Autodesk Inventor part; units mm, degrees
ref_plane "YZ Plane" through (0, 0, 0) normal (1, 0, 0) x (0, 1, 0)
ref_plane "XZ Plane" through (0, 0, 0) normal (0, 1, 0) x (-1, 0, 0)
ref_plane "XY Plane" through (0, 0, 0) normal (0, 0, 1) x (1, 0, 0)
sketch "スケッチ1" plane through (0, 0, 0) normal (0, 0, 1) x (1, 0, 0)
  circle A0 centre (0, 0) radius 3
  circle A1 centre (0, 0) radius 1.25
  dimension "d0" = 6
  dimension "d1" = 2.5
extrude "押し出し1" add sketch "スケッチ1" along normal blind 50 contours A0 | A1
sketch "スケッチ2" plane through (0, 0, 50) normal (0, 0, 1) x (1, 0, 0)
  circle A0 centre (0, 0) radius 3
  circle A1 centre (0, 0) radius 1.25
  dimension "d4" = 2.5
extrude "押し出し2" cut sketch "スケッチ2" against normal blind 5 contours A1
extrude "押し出し3" cut sketch "スケッチ1" along normal blind 5 contours A1
properties part number "50mm" material "アルミニウム 2014-T4"
Geometry check sheet. Reference: the model listing, model coordinates, mm. A direction names the side the tool comes from. Give positions to 0.01 mm unless a question says otherwise; leave off trailing zeros. Write each loop counter-clockwise with the first axis right and the second up, starting at its lowest first coordinate (ties: lowest second). Pieces come first, ordered by that corner, then holes. Notation, with made-up numbers: M 40,-17 L 99,-17 A16 cw 99,-3 Z; hole C 67,21 d3. An arc over 180 degrees is marked long. Answer as CSV lines item,"result". Start each with the question number.
Q1. Section check C-C, the plane z = 10.5. Record the cut outline in (x, y).
Q2. Section check D-D, the plane y = 2.05. Record the cut outline in (x, z), then the cut area to 3 significant figures.
Q3. Material ranges on L1, parallel to Y at x = 0, z = 46.8; L2, parallel to Z at x = 0, y = 0.1; L3, parallel to Y at x = 0.1, z = 12, recorded low to high.
Q4. Release check for a two-part mould opening along Y. For faces 1 (the face through (-3, 0, 25)), 2 (the face through (-0.27, 1.22, 2.46)), 3 (the face through (1, -1, 0)) record: pulls with the +Y half, pulls with the -Y half, needs draft (parallel to the pull), parting line crosses it, or undercut.
Q5. Section check A-A, the plane x = 0. Record the cut outline in (y, z).
Q6. Tool access check on faces 4 (the face through (-0.27, -1.22, 47.54)), 5 (the face through (1, -1, 50)), 6 (the face through (0, 0, 5)). Record the directions out of +Z, -Z, +X, -X, +Y, -Y that give a thin tool (end or side, any length) a straight path to the whole face; none if there is none.
Q7. Go/stop test with flat-tipped pins: pin 1 (2 mm diameter, centred on x = -2, y = -2, fed in from -Z); pin 2 (2 mm diameter, centred on x = 0, y = 0, fed in from +Z). Record where each tip stops, or that it passes through.
Geometry says:
1,outline,"C 0,0 d6"
2,outline,"M -2.19,0 L 2.19,0 L 2.19,50 L -2.19,50 Z"
2,area,"219 mm^2"
3,L1,"-3 to -1.25, 1.25 to 3"
3,L2,"5 to 45"
3,L3,"-3 to 3"
4,face 1,"parting line crosses it"
4,face 2,"undercut"
4,face 3,"needs draft"
5,outline,"M -3,0 L -1.25,0 L -1.25,5 L 1.25,5 L 1.25,0 L 3,0 L 3,50 L 1.25,50 L 1.25,45 L -1.25,45 L -1.25,50 L -3,50 Z"
6,face 4,"+Z"
6,face 5,"+Z, +X, -X, +Y, -Y"
6,face 6,"-Z"
7,pin 1,"z = 0"
7,pin 2,"z = 45"
